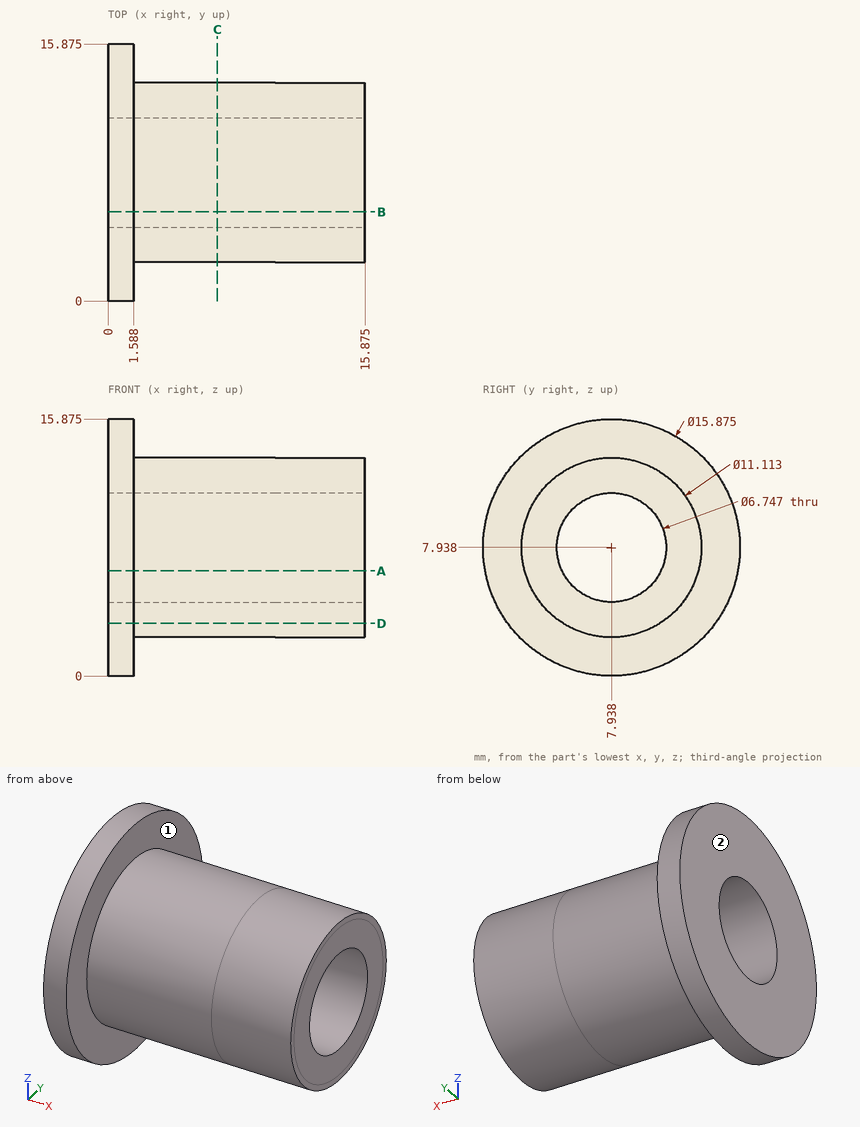
Can you work these out from the drawing? Everything is in mm from the part's minimum corner. A direction names the side the tool comes from. Coordinates: 2 decimals unless noted, no trailing zeros. Loops run counter-clockwise (first coordinate to the right, second up) from the corner with the lowest first, then second, coordinate; pieces in that order, holes last. Notation, with made-up numbers: (4.25, 62) - (21.25, 62) arc R27 cw to (21.25, 91) - close; hole circle Ø5 at (37.5, 37.5). An arc over 180 degrees is marked (long way). Answer as CSV lines item,"result".
Q1. If I drill on L1, parallel to X at y = 13.5, z = 9.5; L2, parallel to Z at x = 3.5, y = 10.25 (1 decimal); L3, parallel to Y at x = 1, z = 5.5 (1 decimal), over which ranges is the centre line in solid material (lowest first)? Write a range as [from, to].
Response:
L1,"[0, 1.59]"
L2,"[2.9, 5.5], [10.4, 13]"
L3,"[0.4, 5.6], [10.3, 15.5]"
Q2. If we section it at D-D, the plane z = 3.25: Write out the boundary of the cut face in (x, y) (1 decimal).
Response:
outline,"(0, 1.5) - (1.6, 1.5) - (1.6, 5) - (15.9, 5) - (15.9, 10.9) - (1.6, 10.9) - (1.6, 14.3) - (0, 14.3) - close"
Q3. If we section it at A-A, the plane z = 6.5: Write out the boundary of the cut face in (x, y) (1 decimal).
Response:
outline,"(0, 0.1) - (1.6, 0.1) - (1.6, 2.6) - (15.9, 2.6) - (15.9, 4.9) - (0, 4.9) - close; (0, 11) - (15.9, 11) - (15.9, 13.3) - (1.6, 13.3) - (1.6, 15.7) - (0, 15.7) - close"
Q4. For pin 1 (1 mm diameter, centred on x = 13, z = 9, fed in from +Y) (1 decimal); pin 2 (8 mm diameter, centred on x = 2.5, y = 13.5, fed in from -Z); pin 3 (4 mm diameter, centred on x = 4, z = 4, fed in from +Y) (1 decimal), each with a flat end and sliding along its axis, tell me the tip position at first contact or that it passes through.
Response:
pin 1,"y = 13.5"
pin 2,"z = 0.18"
pin 3,"y = 13.1"
Q5. For the marked faces 1 and 2, which set-ups out of +Z, -Z, +X, -X, +Y, -Y let a thin tool reach every point of the face, with its end or its side?
Response:
face 1,"+X"
face 2,"+Z, -Z, -X, +Y, -Y"
Q6. If we section it at C-C, the plane x = 6.75: Write out the boundary of the cut face in (y, z).
Response:
outline,"circle Ø11.11 at (7.94, 7.94); hole circle Ø6.75 at (7.94, 7.94)"
Q7. If we section it at B-B, the plane y = 5.5: Write out the boundary of the cut face in (x, z) (1 decimal).
Response:
outline,"(0, 0.4) - (1.6, 0.4) - (1.6, 2.9) - (15.9, 2.9) - (15.9, 5.6) - (0, 5.6) - close; (0, 10.3) - (15.9, 10.3) - (15.9, 12.9) - (1.6, 12.9) - (1.6, 15.5) - (0, 15.5) - close"
